Verification items for the finished model (mm, model axes). A direction names the side the tool comes from. Coordinates: 2 decimals unless noted, no trailing zeros. Order: outer loops, then holes, each group sorted by start corner. A loop starts at its lowest first (then second) coordinate and runs counter-clockwise, first axis right, second up.
Q1. Cross-section at C-C, the plane y = -9.5. Record the boundary of the cut face in (x, z), and give its area (3 significant figures).
Q2. Cross-section at A-A, the plane y = 8.89. Record the boundary of the cut face in (x, z) (3 decimals), and give its area (3 significant figures).
Q3. Cross-section at B-B, the plane z = -0.9. Record the boundary of the cut face in (x, y) (3 decimals), and give its area (3 significant figures).
Q4. Depth check by flat-ended pin: P1, Ø0.7, axis at y = -1.5, z = 0, coming from the -X side. Enter the tip coordinate at first touch or a pass-through.
Q5. Set-up check for faces 1 (the cylindrical face through (1.358, 1.875, -0.022)), 2 (the flat face through (-3.757, -2.912, -0.022)), 3 (the flat face through (12, 0, -1.562)): record each of +Z, -Z, +X, -X, +Y, -Y from which the full face is reachable in a straight line by a thin tool's end or side.
Q6. Thickness scan on line 1 (Y direction, x = 6, z = -0.9); line 2 (Y direction, x = 14.29, z = 0.2); line 3 (Y direction, x = 13, z = 0.55). Record the ranges inside material, lowest first.
Q7. Draft check along Y on faces 4 (the flat face through (9, -16.51, 0)), 5 (the flat face through (-7.62, -10, 0)), 6 (the cylindrical face through (13.085, -4.578, -0.022)). Enter one of: pulls with the +Y half, pulls with the -Y half, needs draft (parallel to the pull), parting line crosses it, or undercut.
Autodesk Fusion 360 part; units mm, degrees
sketch "Sketch1" plane through (0, 0, 0) normal (0, 0, 1) x (1, 0, 0)
  line L0 (-7.62, 16.51) -> (25.4, 16.51)
  line L1 (25.4, 16.51) -> (25.4, -16.51)
  line L2 (25.4, -16.51) -> (-7.62, -16.51)
  circle A0 centre (0, 8.89) radius 3.175
  circle A1 centre (0, -8.89) radius 3.175
  circle A2 centre (13.15, 2.61) radius 0.89
  circle A3 centre (14.29, -0.89) radius 0.89
  circle A4 centre (11.63, -4.12) radius 1.525
  line L3 (-7.62, 3.9468) -> (0, 1.905)
  line L4 (2.7588, 1.27) -> (10.16, 1.27)
  arc A5 (10.16, -1.27) -> (10.16, 1.27) centre (10.16, 0) ccw
  line L5 (10.16, -1.27) -> (2.7588, -1.27)
  arc A6 (0, -1.27) -> (2.7588, -1.27) centre (1.3794, 0) ccw
  line L6 (0, -1.27) -> (0, -1.905)
  line L7 (0, -1.905) -> (-7.62, -3.9468)
  line L8 (-7.62, -16.51) -> (-7.62, -3.9468)
  line L9 (-7.62, 3.9468) -> (-7.62, 16.51)
  line L10 (0, 110) -> (0, -80) construction
  line L11 (11.43, -80) -> (11.43, 100) construction
  line L12 (-90, 0) -> (-86.3571, 0) construction
  line L13 (-86.3571, 0) -> (70, 0) construction
  line L14 (0, 1.905) -> (0, 1.27)
  arc A7 (2.7588, 1.27) -> (0, 1.27) centre (1.3794, 0) ccw
  dimension "d1" = 6.35
  dimension "d2" = 7.62
  dimension "d3" = 7.62
  dimension "d4" = 33.02
  dimension "d5" = 1.27
  dimension "d6" = 19.05
  dimension "d10" = 15
  dimension "d11" = 1.905
  dimension "d12" = 1.905
  dimension "d14" = 7.62
  dimension "d15" = 1.78
  dimension "d16" = 1.78
  dimension "d17" = 3.05
  dimension "d18" = 12.39
  dimension "d19" = 13.77
  dimension "d20" = 11.11
  dimension "d21" = 15.62
  dimension "d22" = 12.25
  dimension "d23" = 13.9
  dimension "d24" = 33.02
  dimension "d26" = 1.875
  dimension "d27" = 15
  dimension "d28" = 2.54
extrude "Extrude1" add sketch "Sketch1" along normal mid plane 3.124
Check values:
1. outline: (-7.62, -1.56) - (-3.12, -1.56) - (-3.12, 1.56) - (-7.62, 1.56) - close; (3.12, -1.56) - (25.4, -1.56) - (25.4, 1.56) - (3.12, 1.56) - close
1. area: 83.7 mm2
2. outline: (-7.62, -1.562) - (-3.175, -1.562) - (-3.175, 1.562) - (-7.62, 1.562) - close; (3.175, -1.562) - (25.4, -1.562) - (25.4, 1.562) - (3.175, 1.562) - close
2. area: 83.3 mm2
3. outline: (-7.62, -16.51) - (25.4, -16.51) - (25.4, 16.51) - (-7.62, 16.51) - (-7.62, 3.947) - (0, 1.905) - (0, 1.27) arc R1.875 cw to (2.759, 1.27) - (10.16, 1.27) arc R1.27 cw to (10.16, -1.27) - (2.759, -1.27) arc R1.875 cw to (0, -1.27) - (0, -1.905) - (-7.62, -3.947) - close; hole circle Ø6.35 at (0, -8.89); hole circle Ø6.35 at (0, 8.89); hole circle Ø3.05 at (11.63, -4.12); hole circle Ø1.78 at (13.15, 2.61); hole circle Ø1.78 at (14.29, -0.89)
3. area: 939 mm2
4. P1: stops at x = 0
5. face 1: +Z, -Z
5. face 2: +Z, -Z, -X
5. face 3: -Z, +X, -X, +Y, -Y
6. line 1: y = -16.51 to -1.27, 1.27 to 16.51
6. line 2: y = -16.51 to -1.78, 0 to 16.51
6. line 3: y = -16.51 to -4.79, -3.45 to 1.73, 3.49 to 16.51
7. face 4: pulls with the -Y half
7. face 5: needs draft
7. face 6: undercut
